```python
from build123d import *

# Parameters (mm, degrees)
F1_DEPTH = 75.039662


with BuildPart() as f1:
    # F0 (on Front) → F1 (new body)
    with BuildSketch(Plane.XZ):
        with BuildLine():
            Line((-32.266583, 20.745724), (-24.850886, 20.745724))
            ThreePointArc((-24.850886, 20.745724), (-27.760783, 28.835463), (-35.157008, 33.218068))
            Line((-35.157008, 33.218068), (-37.550886, 25.612847))
            ThreePointArc((-37.550886, 25.612847), (-33.900721, 24.2737), (-32.266583, 20.745724))
        make_face()
        with BuildLine():
            ThreePointArc((-37.342298, 8.047438), (-28.497183, 11.839521), (-24.850886, 20.745724))
            Line((-24.850886, 20.745724), (-32.266583, 20.745724))
            ThreePointArc((-32.266583, 20.745724), (-32.26337, 20.64145), (-32.262298, 20.537131))
            ThreePointArc((-32.262298, 20.537131), (-33.750196, 16.945029), (-37.342298, 15.457131))
            Line((-37.342298, 15.457131), (-37.342298, 8.047438))
        make_face()
        with BuildLine():
            Line((-37.550886, 25.612847), (-35.157008, 33.218068))
            ThreePointArc((-35.157008, 33.218068), (-45.640625, 30.535828), (-50.250886, 20.745724))
            Line((-50.250886, 20.745724), (-42.418014, 20.745724))
            ThreePointArc((-42.418014, 20.745724), (-40.934399, 24.129236), (-37.550886, 25.612847))
        make_face()
        with BuildLine():
            ThreePointArc((-50.250886, 20.745724), (-46.45709, 11.692022), (-37.342298, 8.047438))
            Line((-37.342298, 8.047438), (-37.342298, 15.457131))
            ThreePointArc((-37.342298, 15.457131), (-41.007408, 17.019551), (-42.418014, 20.745724))
            Line((-42.418014, 20.745724), (-50.250886, 20.745724))
        make_face()
    extrude(amount=-F1_DEPTH)


solid = f1.part
```
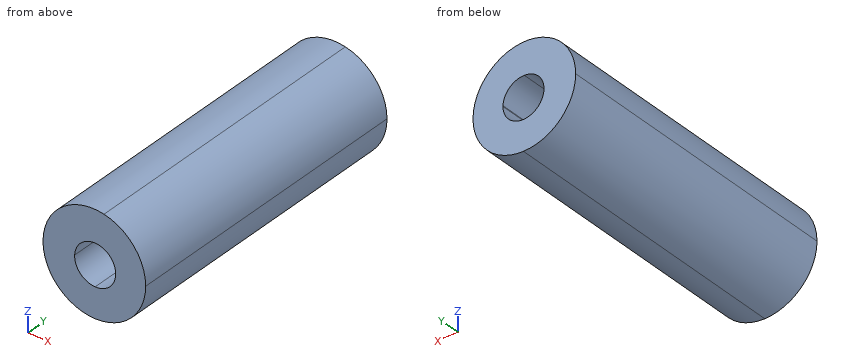
Geometry: final body of the model. Coordinates: model frame, mm. Coordinates: 2 decimals unless noted, no trailing zeros. Order: outer loops, then holes, each group sorted by start corner. A loop starts at its lowest first (then second) coordinate and runs counter-clockwise, first axis right, second up. Notation, with made-up numbers: (63.25, 59) - (110.25, 59) arc R13 cw to (110.25, 80) - close; hole circle Ø3 at (79.25, 51). An arc over 180 degrees is marked (long way). Write each question's results on one line, items separated by ' | '.
1) Section B-B, the plane y = 38. Return loops of the section in (x, z), plus the area to 3 significant figures.
Results list:
outline: (-37.34, 8.05) arc R12.7 ccw to (-24.85, 20.75) arc R12.7 ccw to (-35.16, 33.22) arc R12.7 ccw (long way) to start; hole (-42.42, 20.75) arc R5.08 ccw to (-37.34, 15.46) arc R5.08 ccw to (-32.26, 20.54) arc R5.08 ccw to (-32.27, 20.75) arc R5.08 ccw to (-37.55, 25.61) arc R5.08 ccw to start | area: 426 mm^2
2) Section A-A, the plane x = -39. Return loops of the section in (y, z).
Results list:
outline: (0, 8.13) - (75.04, 8.13) - (75.04, 15.74) - (0, 15.74) - close; (0, 25.34) - (75.04, 25.34) - (75.04, 33.36) - (0, 33.36) - close
3) Section C-C, the plane z = 19.25. Return loops of the section in (x, y).
Results list:
outline: (-50.16, 0) - (-42.26, 0) - (-42.26, 75.04) - (-50.16, 75.04) - close; (-32.43, 0) - (-24.94, 0) - (-24.94, 75.04) - (-32.43, 75.04) - close
4) Pin query (flat end, axial travel): pin 1 (3 mm diameter, centred on y = 63, z = 11, fed in from -X); pin 2 (12 mm diameter, centred on x = -29.5, y = 48.5, fed in from +Z); pin 3 (1.5 mm diameter, centred on y = 59, z = 27.5, fed in from -X). Return the tip coordinate at first contact, or that it passes through.
Results list:
pin 1: x = -47.21 | pin 2: z = 33.28 | pin 3: x = -48.74
5) Line query: line 1 (Z direction, x = -37.25, y = 23); line 2 (X direction, y = 59.5, z = 18.75); line 3 (Z direction, x = -41.5, y = 34). Output: solid intervals per line, ascending. Write a range as from..to.
Results list:
line 1: 8.05..15.46, 25.62..33.44 | line 2: -50.09..-42.1, -32.59..-25.01 | line 3: 8.68..17.62, 23.46..32.82
6) Section D-D, the plane z = 13. Return loops of the section in (x, y), plus the area to 3 significant figures.
Results list:
outline: (-47.62, 0) - (-27.49, 0) - (-27.49, 75.04) - (-47.62, 75.04) - close | area: 1,510 mm^2
